Verification items for this drawing (mm, ordinates from the low corner). Round coordinates to 2 decimals unless told otherwise and drop trailing zeros. Loops run counter-clockwise (first coordinate to the right, second up) from the corner with the lowest first, then second, coordinate; pieces in that order, holes last. Notation, with made-up numbers: (9, 63.25) -> (16, 63.25) arc R14 ccw to (16, 82.25) -> close; hole circle Ø10 at (18.25, 45). An arc over 180 degrees is marked (long way). Use a Markdown table: item, result. Add a question column.
Q1. Material ranges on L1, parallel to X at y = 1.05, z = 12.7 (1 decimal); L2, parallel to Y at x = 12, z = 20; L3, parallel to Z at x = 3.5, y = 5.5, recorded low to high.
Q2. Sectioned sample at A-A, the plane y = 5.75. Enter the section's corners in (x, z), then the cut area to 3 significant figures.
Q3. Gauge pin test, flat ends, axial feed: P1, Ø5, axis at x = 27, z = 15, coming from the +Y side; P2, Ø0.6, axis at x = 6, y = 5, coming from the -Z side; P3, Ø0.6, axis at x = 4, y = 6, coming from the +Z side. Record the tip position at first contact, or that the pin passes through.
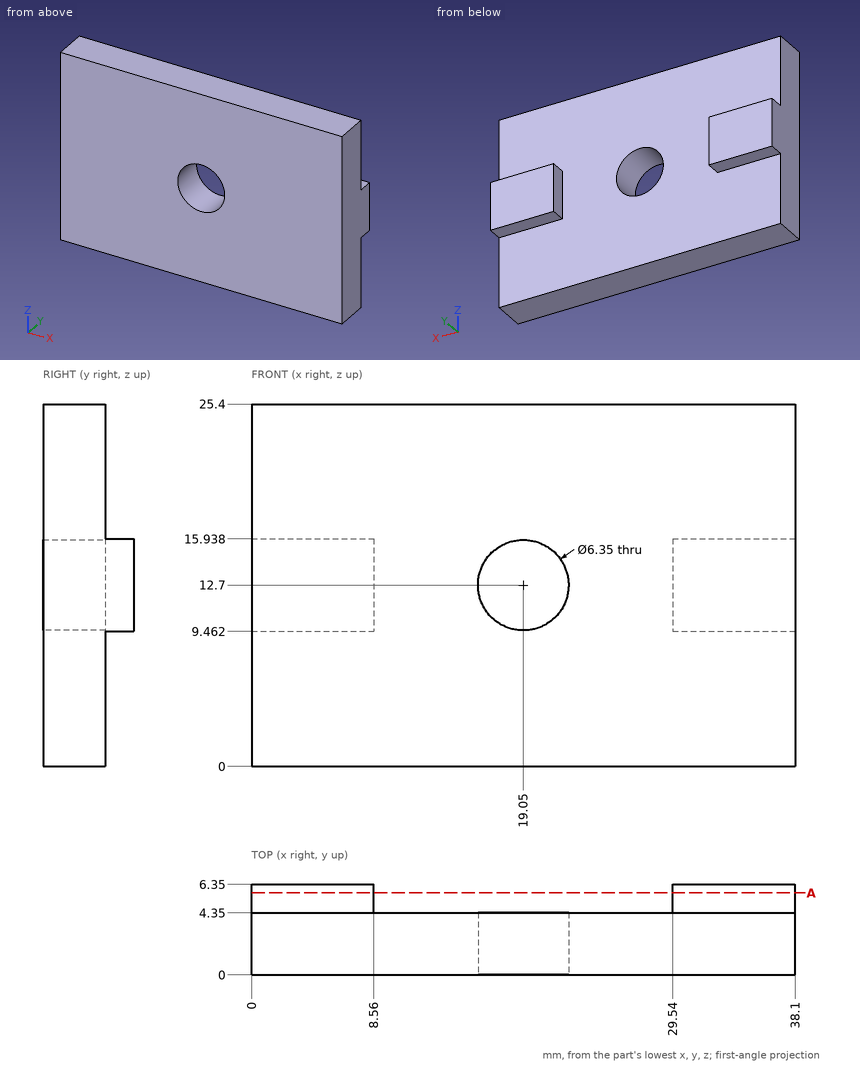
Values:
| question | item | result |
|---|---|---|
| 1 | L1 | 0 to 15.9, 22.2 to 38.1 |
| 1 | L2 | 0 to 4.35 |
| 1 | L3 | 9.46 to 15.94 |
| 2 | outline | (0, 9.46) -> (8.56, 9.46) -> (8.56, 15.94) -> (0, 15.94) -> close; (29.54, 9.46) -> (38.1, 9.46) -> (38.1, 15.94) -> (29.54, 15.94) -> close |
| 2 | area | 111 mm^2 |
| 3 | P1 | y = 4.35 |
| 3 | P2 | z = 9.46 |
| 3 | P3 | z = 15.94 |
